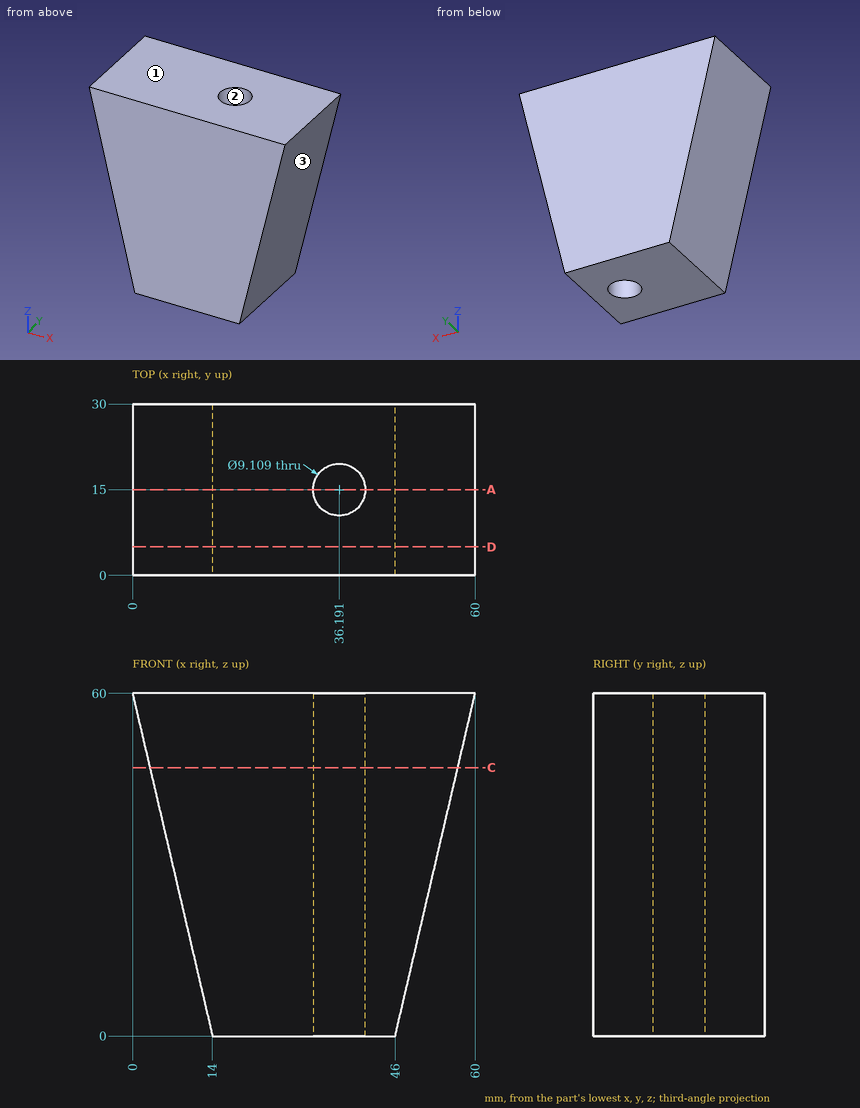
Verification items for this drawing (mm, ordinates from the low corner). Coordinates: 2 decimals unless noted, no trailing zeros. Write each loop counter-clockwise with the first axis right and the second up, starting at its lowest first coordinate (ties: lowest second). Pieces come first, ordered by that corner, then holes. Notation, with made-up numbers: (55, 33) - (106, 33) arc R13 cw to (106, 55) - close; hole circle Ø11 at (63.25, 23.5). An arc over 180 degrees is marked (long way). One line per question, with ' | ' between items.
Item 1: Thickness scan on line 1 (Y direction, x = 32, z = 50.5) (1 decimal); line 2 (X direction, y = 17.75, z = 48.5) (1 decimal); line 3 (Y direction, x = 35, z = 8). Record the ranges inside material, lowest first. Write a range as [from, to].
Determined:
line 1: y = [0, 13.2], [16.8, 30] | line 2: x = [2.7, 32.6], [39.8, 57.3] | line 3: y = [0, 10.6], [19.4, 30]
Item 2: Sectioned sample at C-C on z = 47. Record the boundary of the cut face in (x, y) (1 decimal), plus the area to 3 significant figures.
Determined:
outline: (3, 0) - (57, 0) - (57, 30) - (3, 30) - close; hole circle Ø9.1 at (36.2, 15) | area: 1,550 mm2
Item 3: Sectioned sample at A-A on y = 15. Record the boundary of the cut face in (x, z) (1 decimal).
Determined:
outline: (0, 60) - (14, 0) - (31.6, 0) - (31.6, 60) - close; (40.7, 0) - (46, 0) - (60, 60) - (40.7, 60) - close
Item 4: Sectioned sample at D-D on y = 5. Record the boundary of the cut face in (x, z), plus the area to 3 significant figures.
Determined:
outline: (0, 60) - (14, 0) - (46, 0) - (60, 60) - close | area: 2,760 mm2
Item 5: Gauge pin test, flat ends, axial feed: P1, Ø1.5, axis at y = 20.5, z = 7.5, coming from the +X side (1 decimal); P2, Ø1, axis at y = 4, z = 23, coming from the +X side; P3, Ø12, axis at y = 20.5, z = 11, coming from the -X side. Record the tip position at first contact, or that the pin passes through.
Determined:
P1: stops at x = 47.9 | P2: stops at x = 51.48 | P3: stops at x = 10.03
Item 6: Mould release check, pull along X, two halves, no side actions. Record for the marked faces 1, 2 and 3: pulls with the +X half, pulls with the -X half, needs draft (parallel to the pull), parting line crosses it, or undercut.
Determined:
face 1: needs draft | face 2: undercut | face 3: pulls with the +X half
